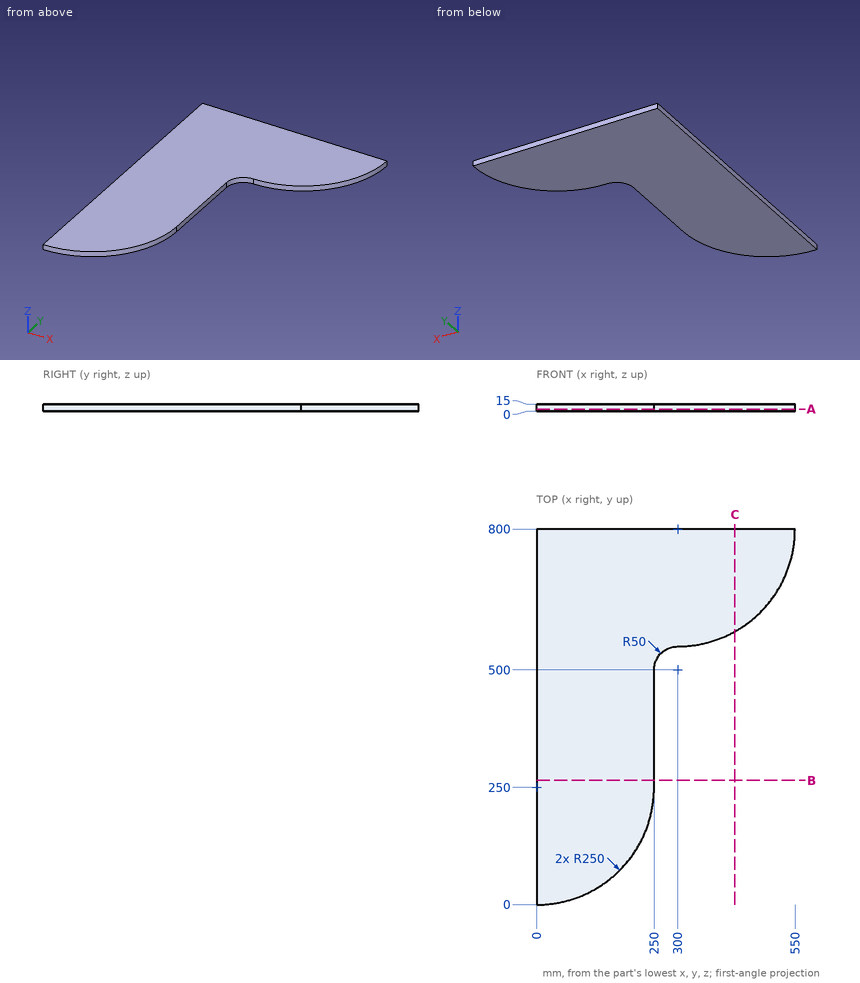
Check sheet for the drawn part. Datum: minimum x, y, z corner. Units: mm. Give positions to 0.01 mm unless a question says otherwise; leave off trailing zeros. Write each loop counter-clockwise with the first axis right and the second up, starting at its lowest first coordinate (ties: lowest second). Pieces come first, ordered by that corner, then holes.
(1) Cross-section at C-C (x = 422). Enter the section's corners in (y, z).
(2) Gauge pin test, flat ends, axial feed: pin 1 (6 mm diameter, centred on x = 197, z = 7.5, fed in from -Y); pin 2 (4.5 mm diameter, centred on y = 410.5, z = 7, fed in from +X). Record the tip position at first contact, or that the pin passes through.
(3) Material ranges on line 1 (X direction, y = 302.5, z = 9.5); line 2 (Y direction, x = 45, z = 3.5); line 3 (Y direction, x = 393.5, z = 0.75), recorded low to high.
(4) Cross-section at B-B (y = 265). Enter the section's corners in (x, z).
(5) Cross-section at A-A (z = 4.25). Enter the section's corners in (x, y), plus the area to 3 significant figures.
Worked out:
1. outline: (581.79, 0) - (800, 0) - (800, 15) - (581.79, 15) - close
2. pin 1: stops at y = 92.32
2. pin 2: stops at x = 250
3. line 1: x = 0 to 250
3. line 2: y = 4.08 to 800
3. line 3: y = 568.14 to 800
4. outline: (0, 0) - (250, 0) - (250, 15) - (0, 15) - close
5. outline: (0, 0) arc R250 ccw to (250, 250) - (250, 500) arc R50 cw to (300, 550) arc R250 ccw to (550, 800) - (0, 800) - close
5. area: 249,000 mm2
